from build123d import *

# Parameters (mm, degrees)
SKETCH1_W                = 25
SKETCH1_H                = 38
SKETCH1_W_2              = 16.5
SKETCH1_H_2              = 1.4
BOSS_EXTRUDE1_DEPTH      = 2
SKETCH1_3_W              = 16.5
SKETCH1_3_H              = 1.4
BOSS_EXTRUDE2_DEPTH      = 5.5
BOSS_EXTRUDE3_DEPTH      = 3
BOSS_EXTRUDE3_DEPTH_BACK = 3


with BuildPart() as part:
    # Sketch1 → Boss-Extrude1 (new body)
    with BuildSketch(Plane(origin=(0, 0, 0), x_dir=(1, 0, 0), z_dir=(0, 1, 0))):
        Rectangle(SKETCH1_W, SKETCH1_H)
        with Locations((0, -17.2)):
            Rectangle(SKETCH1_W_2, SKETCH1_H_2, mode=Mode.SUBTRACT)
        with Locations((0, 17.2)):
            Rectangle(SKETCH1_W_2, SKETCH1_H_2, mode=Mode.SUBTRACT)
    extrude(amount=BOSS_EXTRUDE1_DEPTH)

    # Sketch1<3> → Boss-Extrude2 (add)
    with BuildSketch(Plane(origin=(0, 0, 0), x_dir=(1, 0, 0), z_dir=(0, 1, 0))):
        Polygon((-14, -1.5), (-12.5, -3), (-12.5, 3), (-14, 1.5), align=None)
        Polygon((12.5, 3), (12.5, -3), (14, -1.5), (14, 1.5), align=None)
        with Locations((0, 17.2)):
            Rectangle(SKETCH1_3_W, SKETCH1_3_H)
        with Locations((0, -17.2)):
            Rectangle(SKETCH1_3_W, SKETCH1_3_H)
    extrude(amount=BOSS_EXTRUDE2_DEPTH)

    # Sketch2 → Boss-Extrude3 (add, two sides: drawn at the far end of the back side and taken through both)
    with BuildSketch(Plane.XY.offset(-BOSS_EXTRUDE3_DEPTH_BACK)):
        Polygon((12.5, 5.5), (11.5, 4.5), (12.5, 4.5), align=None)
        Polygon((-11.5, 4.5), (-12.5, 4.5), (-12.5, 5.5), align=None)
    extrude(amount=BOSS_EXTRUDE3_DEPTH + BOSS_EXTRUDE3_DEPTH_BACK)


solid = part.part
For this review, take the finished solid that the model builds, in its own axes (mm). A direction names the side the tool comes from. Round coordinates to 2 decimals unless told otherwise and drop trailing zeros. Write each loop counter-clockwise with the first axis right and the second up, starting at its lowest first coordinate (ties: lowest second). Pieces come first, ordered by that corner, then holes. Notation, with made-up numbers: M 40,-33 L 48,-33 A9 ccw 48,-16 Z; hole C 25.25,14 d7. An arc over 180 degrees is marked long. Write item = value, one per line. Start each with the question number.
(1) For line 1 along Z through (x, y) = (-7, 2.65); line 2 along Y through (x, z) = (-7.75, 14.5); line 3 along X through (y, z) = (2.55, 17.5), list the stretches that pass through material, from the lowest coordinate up.
(2) For faces 5 (the face through (-12, 4.5, 0)), 6 (the face through (12.2, 4.8, -3)), 7 (the face through (0, 4, 16.5)), 8 (the face through (-12.2, 4.8, 3)), 9 (the face through (-8.25, 4, -17)), list the 3-axis set-ups (+Z, -Z, +X, -X, +Y, -Y) from which the entire face can be reached by the end or side of a thin tool; tool diameter is ignored.
(3) We need section A-A (y = 3). Give the boundary of the cut face in (x, z).
(4) We need section C-C (z = 2). Give the boundary of the cut face in (x, y), then the cut area to 3 significant figures.
(5) The part is to be moulded in two halves that separate along X. For faces 1 (the face through (12, 4.5, 0)), 2 (the face through (-12.5, 3, 0)), 3 (the face through (8.25, 4, -17)), 4 (the face through (0, 5.5, 17)), say which applies: +X half, -X half, draft (parallel to the pull), parting line (faces both ways), or undercut.
(6) We need section B-B (x = -0.25). Give the boundary of the cut face in (y, z).
(7) Clearance check with flat-ended pins moving along their axes: pin 1 Ø1 at (y, z) = (0.5, -14) entering from +X; pin 2 Ø3 at (x, y) = (-2.5, 4) entering from +Z; pin 3 Ø4 at (x, z) = (0, 4.5) entering from +Y. State where each tip first meets the part, or that it passes through.
(8) We need section D-D (z = -12). Give the boundary of the cut face in (x, y).
Results found:
q1.line_1 = -17.9 to -16.5, 16.5 to 17.9
q1.line_2 = 0 to 2
q1.line_3 = -8.25 to 8.25
q2.face_5 = +Z, -Z
q2.face_6 = -Z, +X, -X, +Y
q2.face_7 = +X, -X, +Y
q2.face_8 = +Z, +X, -X, +Y
q2.face_9 = +Z, -Z, -X, +Y
q3.outline = M -14,-1.5 L -12.5,-3 L -12.5,3 L -14,1.5 Z; M -8.25,-17.9 L 8.25,-17.9 L 8.25,-16.5 L -8.25,-16.5 Z; M -8.25,16.5 L 8.25,16.5 L 8.25,17.9 L -8.25,17.9 Z; M 12.5,-3 L 14,-1.5 L 14,1.5 L 12.5,3 Z
q4.outline = M -13.5,0 L 13.5,0 L 13.5,5.5 L 12.5,5.5 L 11.5,4.5 L 12.5,4.5 L 12.5,2 L -12.5,2 L -12.5,4.5 L -11.5,4.5 L -12.5,5.5 L -13.5,5.5 Z
q4.area = 62.0 mm²
q5.face_1 = undercut
q5.face_2 = undercut
q5.face_3 = +X half
q5.face_4 = draft
q6.outline = M 0,-19 L 2,-19 L 2,-17.9 L 5.5,-17.9 L 5.5,-16.5 L 2,-16.5 L 2,16.5 L 5.5,16.5 L 5.5,17.9 L 2,17.9 L 2,19 L 0,19 Z
q7.pin_1 = 12.5
q7.pin_2 = 17.9
q7.pin_3 = 2
q8.outline = M -12.5,0 L 12.5,0 L 12.5,2 L -12.5,2 Z
